Geometry: final body of the model. Coordinates: model frame, mm. A direction names the side the tool comes from. Coordinates: 2 decimals unless noted, no trailing zeros. Order: outer loops, then holes, each group sorted by start corner. A loop starts at its lowest first (then second) coordinate and runs counter-clockwise, first axis right, second up. Notation, with made-up numbers: M 35,-19 L 88,-19 A11 cw 88,-10 Z; hole C 15.25,-37.75 d3. An arc over 180 degrees is marked long. Use CSV: the item, a comma, the result in double quotes. Start each with the question number.
Q1. Section query B-B, the plane x = -12.25. State how many separate pieces and enclosed holes the cut face has, and give its area (3 significant figures).
Q2. Section query A-A, the plane y = 21.59. Output: boundary loops of the cut face in (x, z) (3 decimals).
Q3. Mould query, pull axis Y, two halves, no side actions, for faces 4 (the face through (-8.357, 31.25, -18.47)), 5 (the face through (-7, 6.35, -16)), 6 (the face through (-6, 44.45, -18)), 7 (the face through (-7.48, 47.58, -20.14)). Classes: +Y half, -Y half, draft (parallel to the pull), parting line (faces both ways), or undercut.
Q4. Access query for faces 1 (the face through (-4, 50.8, -17)), 2 (the face through (-4.68, 3.22, -16.22)), 3 (the face through (-1.549, 35, -17)). Directions: +Z, -Z, +X, -X, +Y, -Y. A direction counts if a zero-diameter tool reaches every point of the face in a straight line with its end or side. Return the directions, or none.
Q5. First-contact query: P1, Ø4.5, axis at x = -7.37, z = -17.46, coming from the +Y side. Flat tip, straight axial feed; report the tip coordinate or a pass-through.
Q6. Ray query, probe 1 along Y at (x, z) = (-12, -3.5); probe 2 along Z at (x, y) = (-12, 5) (3 decimals); probe 3 along Z at (x, y) = (-11.25, 4) (3 decimals). Return the intervals inside material, ascending.
Q7. Section query C-C, the plane x = -4. Output: boundary loops of the cut face in (y, z) (3 decimals), and give its area (3 significant figures).
Autodesk Inventor part; units mm, degrees
ref_plane "YZ Plane" through (0, 0, 0) normal (1, 0, 0) x (0, 1, 0)
ref_plane "XZ Plane" through (0, 0, 0) normal (0, 1, 0) x (-1, 0, 0)
ref_plane "XY Plane" through (0, 0, 0) normal (0, 0, 1) x (1, 0, 0)
sketch "Sketch1" plane through (0, 0, 0) normal (0, 1, 0) x (-1, 0, 0)
  line L0 (0, 0) -> (14.732, 0)
  line L1 (14.732, 0) -> (14.732, -34.925)
  line L2 (14.732, -34.925) -> (0, -34.925)
  line L3 (0, -34.925) -> (0, 0)
  dimension "BlockW" = 14.732
  dimension "BlockL" = 34.925
extrude "Extrusion1" add sketch "Sketch1" along normal blind 50.8
sketch "Sketch3" plane through (0, 0, 0) normal (1, 0, 0) x (0, 0, -1)
  line L0 (0, 0) -> (17.4752, 0)
  line L1 (0, 21.59) -> (0, 0)
  circle A0 centre (17.4752, 21.59) radius 9.525
  circle A1 centre (17.4752, 21.59) radius 12.954
  circle A2 centre (17.4752, 21.59) radius 16.129
  line L2 (4.318, 21.59) -> (21.59, 21.59) construction
  point P0 (4.318, 38.862)
  dimension "d15" = 19.05
  dimension "d16" = 25.908
  dimension "d17" = 32.258
hole "Hole2" at (0, 38.862, -4.318) direction (-1, 0, 0) diameter 3.302 depth 10.16
pattern_linear "Rectangular Pattern1" count 2 spacing 26.289 along (0, 0, -1) count 2 spacing 34.544 along (0, -1, 0) of "Hole2"
extrude "Extrusion2" cut sketch "Sketch3" against normal through all contours A0
extrude "Extrusion3" cut sketch "Sketch3" against normal blind 6.3754 contours A1
extrude "Extrusion4" cut sketch "Sketch3" against normal blind 1.5494 contours A2
sketch "Sketch4" plane through (-14.732, 0, -34.925) normal (-1, 0, 0) x (0, 0, 1)
  line L0 (0, 0) -> (17.4752, 0)
  line L1 (17.4752, 21.59) -> (0, 21.59)
  line L2 (0, 21.59) -> (0, 0)
  circle A0 centre (17.4752, 21.59) radius 9.525
  circle A1 centre (17.4752, 21.59) radius 12.954
  circle A2 centre (17.4752, 21.59) radius 16.129
  line L3 (17.4752, 21.59) -> (30.6197, 21.59)
  line L4 (30.6197, 21.59) -> (30.6197, 38.862)
  line L5 (30.6197, 38.862) -> (17.4752, 38.862)
  line L6 (17.4752, 38.862) -> (17.4752, 21.59)
  point P0 (34.925, 0)
  dimension "d24" = 17.4752
  dimension "d25" = 21.59
  dimension "d26" = 19.05
  dimension "d28" = 32.258
  dimension "d57" = 13.1445
  dimension "d58" = 17.272
extrude "Extrusion5" cut sketch "Sketch4" against normal blind 6.3754 contours A0 L3 A1 L1 | L1 A1 L6 A0 | A0 L6 A1 L3
extrude "Extrusion6" cut sketch "Sketch4" against normal blind 1.5494 contours A1 L3 L4 A2 L1 | L1 A2 L6 A1 | A1 L6 A2 L4 L3
hole "Hole3" at (-14.732, 38.862, -4.3053) direction (1, 0, 0) diameter 3.302 depth 10.16
pattern_linear "Rectangular Pattern2" count 2 spacing 26.289 along (0, 0, -1) count 2 spacing 34.544 along (0, -1, 0) of "Hole3"
sketch "Sketch5" plane through (0, 50.8, 0) normal (0, 1, 0) x (1, 0, 0)
  line L0 (-14.732, 0) -> (0, 0)
  line L1 (-7.366, 0) -> (-7.366, 34.925)
  line L2 (0, 34.925) -> (-14.732, 34.925)
  line L3 (-7.366, 34.925) -> (-7.366, 17.4625)
hole "Hole4" at (-7.366, 50.8, -17.4625) direction (0, -1, 0) diameter 1.5875 end through all
hole "Hole5" at (-7.366, 50.8, -17.4625) direction (0, -1, 0) diameter 5.3594 depth 6.35
sketch "Sketch7" plane through (0, 0, 0) normal (0, -1, 0) x (1, 0, 0)
  point P0 (0, 0)
  point P1 (-7.2944, -16.8018)
hole "Hole6" at (-7.2944, 0, -16.8018) direction (0, 1, 0) diameter 5.3594 depth 6.35
properties part number "FlowTiCell"
Responses:
1,separate pieces,"2"
1,enclosed holes,"5"
1,area,"1,210 mm²"
2,outline,"M -14.732,-34.925 L 0,-34.925 L 0,-33.604 L -1.549,-33.604 L -1.549,-30.429 L -6.375,-30.429 L -6.375,-27 L -8.357,-27 L -8.357,-30.404 L -13.183,-30.404 L -13.183,-33.579 L -14.732,-33.579 Z; M -14.732,-7.95 L -6.375,-7.95 L -6.375,-4.521 L -1.549,-4.521 L -1.549,-1.346 L 0,-1.346 L 0,0 L -14.732,0 L -14.732,-1.321 L -13.183,-1.321 L -13.183,-4.496 L -8.357,-4.496 L -8.357,-7.925 L -14.732,-7.925 Z"
3,face 4,"undercut"
3,face 5,"-Y half"
3,face 6,"+Y half"
3,face 7,"draft"
4,face 1,"+Z, -Z, +X, -X, +Y"
4,face 2,"-Y"
4,face 3,"+X"
5,P1,"stops at y = 44.45"
6,probe 1,"y = 0 to 2.88, 5.76 to 37.42, 40.3 to 50.8"
6,probe 2,"z = -34.925 to -32.098, -29.091 to -5.809, -2.802 to 0"
6,probe 3,"z = -34.925 to -32.214, -28.974 to -5.925, -2.685 to 0"
7,outline,"M 0,-34.925 L 50.8,-34.925 L 50.8,0 L 0,0 Z; hole C 4.318,-30.607 d3.302; hole C 4.318,-4.318 d3.302; hole C 21.59,-17.475 d25.908; hole C 38.862,-30.607 d3.302; hole C 38.862,-4.318 d3.302"
7,area,"1,210 mm²"
